Check sheet for the modelled part. Datum: model origin and axes. Units: mm. Face numbers are marked on the shaded views. Coordinates: 2 decimals unless noted, no trailing zeros. Loops run counter-clockwise (first coordinate to the right, second up) from the corner with the lowest first, then second, coordinate; pieces in that order, holes last. Notation, with made-up numbers: M -2.5,-8.5 L 7.5,-8.5 A30 cw 7.5,22.5 Z; hole C 81,39.25 d1. An arc over 180 degrees is marked long. Answer in a Markdown table with one row per item. Add a question column.
```python
from build123d import *

# Parameters (mm, degrees)
SKETCH1_W           = 127
SKETCH1_H           = 127
BOSS_EXTRUDE1_DEPTH = 12.7
SHELL1_T            = -6.35
SCALE1_SCALE        = 0.5
SKETCH2_R           = 0.79375
CUT_EXTRUDE2_DEPTH  = 69.465251223


with BuildPart() as part:
    # Sketch1 → Boss-Extrude1 (new body)
    with BuildSketch(Plane(origin=(0, 0, 0), x_dir=(1, 0, 0), z_dir=(0, 1, 0))):
        Rectangle(SKETCH1_W, SKETCH1_H)
    extrude(amount=BOSS_EXTRUDE1_DEPTH)

    # Shell1
    shell1_openings = [part.faces().sort_by_distance(p)[0] for p in [
        (0, 0, 0),
    ]]
    offset(amount=SHELL1_T, openings=shell1_openings, kind=Kind.INTERSECTION)


with BuildPart() as part_1:
    # Scale1: scaled about (0, 0, 0)
    add(part.part.scale(SCALE1_SCALE))

    # Sketch2 → Cut-Extrude2 (cut, through all)
    with BuildSketch(Plane(origin=(0, 0, 28.575), x_dir=(-1, 0, 0), z_dir=(0, 0, -1))):
        with Locations((0, 1.5875)):
            Circle(SKETCH2_R)
    extrude(amount=-CUT_EXTRUDE2_DEPTH, mode=Mode.SUBTRACT)


solid = part_1.part
```
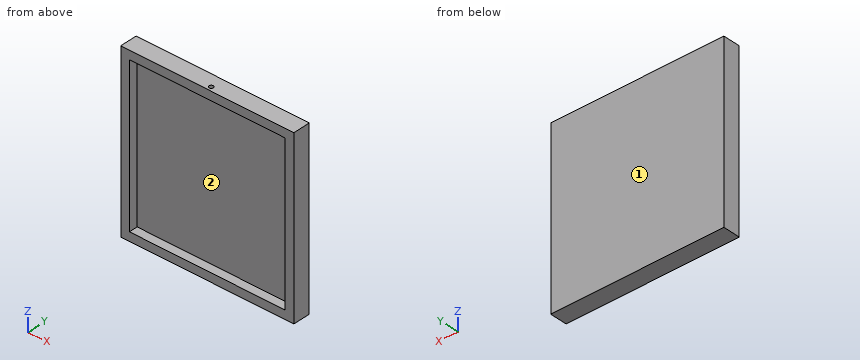
Q1. Cross-section at B-B (z = 27.5). Record the cut outline in (x, y) (3 decimals).
Q2. Mould release check, pull along X, two halves, no side actions. Record for the marked faces 1 and 2: released by +X, released by -X, zero draft, split by the parting line, or undercut.
Q3. Go/stop test with flat-tipped pins: pin 1 (2 mm diameter, centred on x = 0, y = 1.59, fed in from +Z); pin 2 (5 mm diameter, centred on x = 24.5, z = -24.5, fed in from -Y) (3 decimals). Record where each tip stops, or that it passes through.
Q4. Cross-section at C-C (x = -21). Record the cut outline in (y, z) (3 decimals), plus the area to 3 significant figures.
Q5. Thickness scan on L1, parallel to Z at x = 25, y = 2.5 (3 decimals); L2, parallel to Y at x = 0, z = 30.1. Record the ranges inside material, lowest first.
Q6. Cross-section at A-A (x = 0). Record the cut outline in (y, z) (3 decimals), plus the area to 3 significant figures.
Answer key:
| question | item | result |
|---|---|---|
| 1 | outline | M -31.75,0 L -28.575,0 L -28.575,3.175 L 28.575,3.175 L 28.575,0 L 31.75,0 L 31.75,6.35 L -31.75,6.35 Z |
| 2 | face 1 | zero draft |
| 2 | face 2 | undercut |
| 3 | pin 1 | z = 31.75 |
| 3 | pin 2 | y = 3.175 |
| 4 | outline | M 0,-31.75 L 6.35,-31.75 L 6.35,31.75 L 0,31.75 L 0,28.575 L 3.175,28.575 L 3.175,-28.575 L 0,-28.575 Z |
| 4 | area | 222 mm^2 |
| 5 | L1 | -31.75 to -28.575, 28.575 to 31.75 |
| 5 | L2 | 0 to 0.79, 2.38 to 6.35 |
| 6 | outline | M 0,-31.75 L 6.35,-31.75 L 6.35,31.75 L 2.381,31.75 L 2.381,28.575 L 3.175,28.575 L 3.175,-28.575 L 0,-28.575 Z; M 0,28.575 L 0.794,28.575 L 0.794,31.75 L 0,31.75 Z |
| 6 | area | 217 mm^2 |
